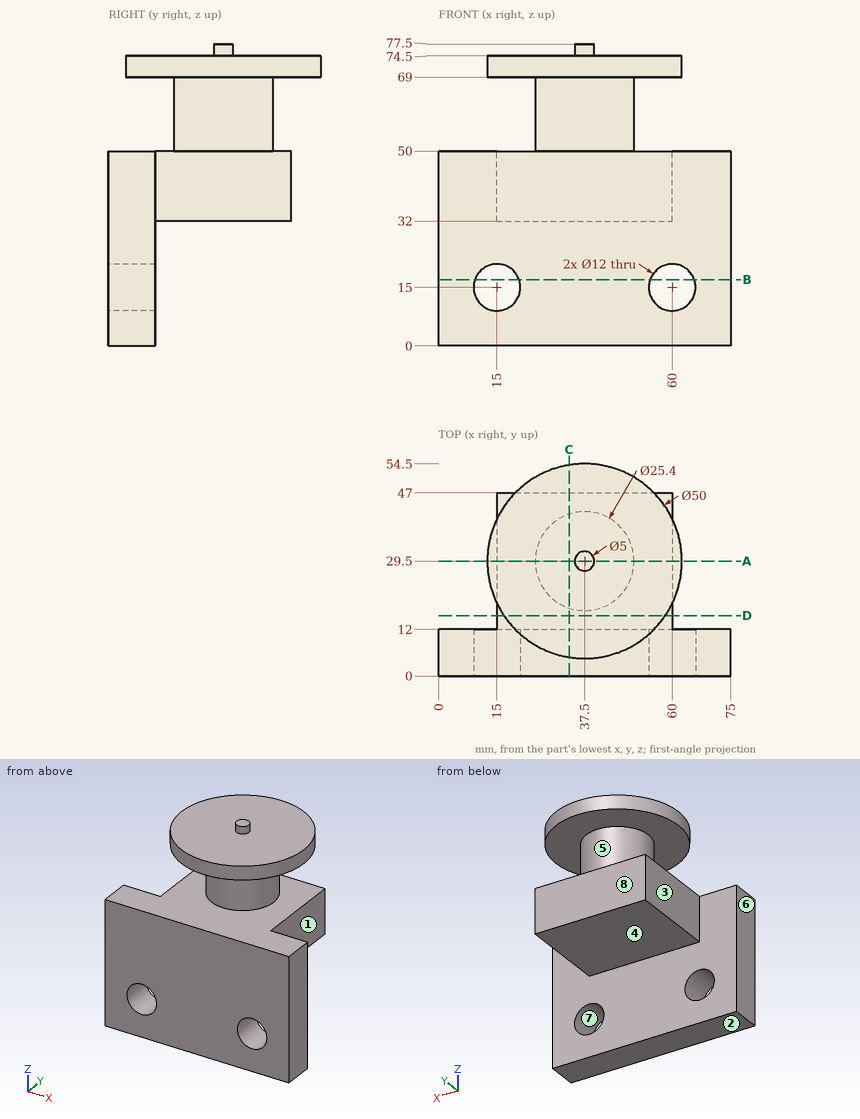
Can you work these out from the drawing? Everything is in mm from the part's minimum corner. A direction names the side the tool comes from. Coordinates: 2 decimals unless noted, no trailing zeros. Write each loop counter-clockwise with the first axis right and the second up, starting at its lowest first coordinate (ties: lowest second). Pieces come first, ordered by that corner, then holes. Notation, with made-up numbers: (25.25, -21) - (67.25, -21) arc R25 ccw to (67.25, 0) - close; hole circle Ø7 at (51.25, 40). An arc over 180 degrees is marked (long way). One line per item, written item: value.
1) Suppose I cut it at B-B on z = 17. Write out the boundary of the cut face in (x, y), and give its area (3 significant figures).
Model answer:
outline: (0, 0) - (9.34, 0) - (9.34, 12) - (0, 12) - close; (20.66, 0) - (54.34, 0) - (54.34, 12) - (20.66, 12) - close; (65.66, 0) - (75, 0) - (75, 12) - (65.66, 12) - close
area: 628 mm²
2) We'd pull the mould along X, two halves only. Please class the marked faces 6, 7 and 8: pulls with the +X half, pulls with the -X half, needs draft (parallel to the pull), parting line crosses it, or undercut.
Model answer:
face 6: pulls with the -X half
face 7: undercut
face 8: needs draft
3) Suppose I cut it at D-D on y = 15.5. Write out the boundary of the cut face in (x, z), and give its area (3 significant figures).
Model answer:
outline: (15, 32) - (60, 32) - (60, 50) - (15, 50) - close; (16.79, 69) - (58.21, 69) - (58.21, 74.5) - (16.79, 74.5) - close
area: 1,040 mm²
4) Suppose I cut it at A-A on y = 29.5. Write out the boundary of the cut face in (x, z), and give its area (3 significant figures).
Model answer:
outline: (12.5, 69) - (24.8, 69) - (24.8, 50) - (15, 50) - (15, 32) - (60, 32) - (60, 50) - (50.2, 50) - (50.2, 69) - (62.5, 69) - (62.5, 74.5) - (40, 74.5) - (40, 77.5) - (35, 77.5) - (35, 74.5) - (12.5, 74.5) - close
area: 1,580 mm²
5) On a 3-axis mill with a long thin cutter (end or side, diameter ignored), from which of +Z, -Z, +X, -X, +Y, -Y can I reach the whole of each face in a straight line? I mean the marked faces 1, 2, 3, 4 and 5. Say none if no direction works.
Model answer:
face 1: -Z, +X, +Y
face 2: -Z, +X, -X, +Y, -Y
face 3: -Z, -X, +Y
face 4: -Z, +X, -X, +Y
face 5: none
6) I need wall thicknesses on line 1 along Z through (x, y) = (15, 2); line 2 along Z through (x, y) = (20.5, 28); line 3 along X through (y, z) = (44.5, 43.5). Which ranges of each line are inside material? Lowest first, please.
Model answer:
line 1: z = 0 to 9, 21 to 50
line 2: z = 32 to 50, 69 to 74.5
line 3: x = 15 to 60
7) Suppose I cut it at C-C on x = 33.5. Write out the boundary of the cut face in (y, z), and give its area (3 significant figures).
Model answer:
outline: (0, 0) - (12, 0) - (12, 32) - (47, 32) - (47, 50) - (41.55, 50) - (41.55, 69) - (54.18, 69) - (54.18, 74.5) - (4.82, 74.5) - (4.82, 69) - (17.45, 69) - (17.45, 50) - (0, 50) - close
area: 1,960 mm²
8) I'm going to push flat-ended pins straight in: P1, Ø5, axis at x = 23, z = 10, coming from the +Y side; P2, Ø14.5, axis at y = 26, z = 42.5, coming from the +X side; P3, Ø5.5, axis at y = 37.5, z = 40, coming from the -X side; P4, Ø9.5, axis at x = 60, z = 15, coming from the -Y side. Where does each tip first touch, or does it pass through?
Model answer:
P1: stops at y = 12
P2: stops at x = 60
P3: stops at x = 15
P4: passes through
